Autodesk Inventor part; units mm, degrees
ref_plane "YZ Plane" through (0, 0, 0) normal (1, 0, 0) x (0, 1, 0)
ref_plane "XZ Plane" through (0, 0, 0) normal (0, 1, 0) x (-1, 0, 0)
ref_plane "XY Plane" through (0, 0, 0) normal (0, 0, 1) x (1, 0, 0)
sketch "Sketch1" plane through (0, 0, 0) normal (0, 0, 1) x (1, 0, 0)
  line L0 (-1.5, 81) -> (1.5, 81)
  line L1 (1.5, 81) -> (1.5, 86)
  line L2 (-1.5, 86) -> (1.5, 86)
  line L3 (-1.5, 86) -> (-1.5, 81)
  arc A0 (-53.4049, -82.5) -> (-44.7446, -87.5) centre (-44.7446, -77.5) ccw
  line L4 (-44.7446, -87.5) -> (44.7446, -87.5)
  arc A1 (44.7446, -87.5) -> (53.4049, -82.5) centre (44.7446, -77.5) ccw
  line L5 (53.4049, -82.5) -> (98.1495, -5)
  arc A2 (98.1495, -5) -> (98.1495, 5) centre (89.4893, 0) ccw
  line L6 (98.1495, 5) -> (53.4049, 82.5)
  arc A3 (53.4049, 82.5) -> (44.7446, 87.5) centre (44.7446, 77.5) ccw
  line L7 (44.7446, 87.5) -> (-44.7446, 87.5)
  arc A4 (-44.7446, 87.5) -> (-53.4049, 82.5) centre (-44.7446, 77.5) ccw
  line L8 (-53.4049, 82.5) -> (-98.1495, 5)
  arc A5 (-98.1495, 5) -> (-98.1495, -5) centre (-89.4893, 0) ccw
  line L9 (-98.1495, -5) -> (-53.4049, -82.5)
  line L10 (-50.8068, -84) -> (-98.1495, -2)
  arc A6 (-98.1495, 2) -> (-98.1495, -2) centre (-94.6854, 0) ccw
  line L11 (-98.1495, 2) -> (-50.8068, 84)
  arc A7 (-47.3427, 86) -> (-50.8068, 84) centre (-47.3427, 82) ccw
  line L12 (-47.3427, 86) -> (47.3427, 86)
  arc A8 (50.8068, 84) -> (47.3427, 86) centre (47.3427, 82) ccw
  line L13 (50.8068, 84) -> (98.1495, 2)
  arc A9 (98.1495, -2) -> (98.1495, 2) centre (94.6854, 0) ccw
  line L14 (98.1495, -2) -> (50.8068, -84)
  arc A10 (47.3427, -86) -> (50.8068, -84) centre (47.3427, -82) ccw
  line L15 (47.3427, -86) -> (-47.3427, -86)
  arc A11 (-50.8068, -84) -> (-47.3427, -86) centre (-47.3427, -82) ccw
  line L16 (47.3427, 89) -> (-47.3427, 89)
  line L17 (1.5, 94) -> (-1.5, 94)
  line L18 (-1.5, 94) -> (-1.5, 89)
  line L19 (1.5, 89) -> (-1.5, 89)
  line L20 (1.5, 89) -> (1.5, 94)
  line L21 (1.5, 97) -> (1.5, 94)
  line L22 (-1.5, 97) -> (1.5, 97)
  line L23 (-1.5, 94) -> (-1.5, 97)
  line L24 (1.5, 94) -> (-1.5, 94)
  line L25 (-1.5, 78) -> (-1.5, 81)
  line L26 (1.5, 78) -> (-1.5, 78)
  line L27 (1.5, 81) -> (1.5, 78)
  line L28 (-1.5, 81) -> (1.5, 81)
  line L29 (-11.5, 89) -> (11.5, 89)
  line L30 (11.5, 89) -> (11.5, 86)
  line L31 (11.5, 86) -> (-11.5, 86)
  line L32 (-11.5, 86) -> (-11.5, 89)
  line L33 (1.5, 92) -> (1.5, 83)
  line L34 (-1.5, 83) -> (-1.5, 92)
  line L35 (1.5, 92) -> (-1.5, 92)
  line L36 (1.5, 83) -> (-1.5, 83)
  point P0 (0, 0)
  dimension "d0" = 10
  dimension "d1" = 10
  dimension "d14" = 3
  dimension "d15" = 3
extrude "Extrusion1" add sketch "Sketch1" along normal blind 4 contours L3 L36 L1 L0 | L3 L2 L1 L36 | L34 L7 L33 L2 | L12 L32 L7 L34 | L33 L7 L30 L12 | L34 L16 L33 L7 | L7 L32 L16 L34 | L33 L16 L30 L7 | L18 L35 L20 L16 | L18 L17 L20 L35
sketch "Sketch2" plane through (0, 0, 4) normal (0, 0, 1) x (1, 0, 0)
  line L0 (1.5, 81) -> (1.5, 86)
  line L1 (1.5, 86) -> (11.5, 86)
  line L2 (11.5, 86) -> (11.5, 89)
  line L3 (11.5, 89) -> (1.5, 89)
  line L4 (1.5, 89) -> (1.5, 94)
  line L5 (-1.5, 94) -> (-1.5, 89)
  line L6 (-1.5, 89) -> (-11.5, 89)
  line L7 (-11.5, 89) -> (-11.5, 86)
  line L8 (-11.5, 86) -> (-1.5, 86)
  line L9 (-1.5, 86) -> (-1.5, 81)
  line L10 (-1.5, 81) -> (1.5, 81)
  line L11 (1.5, 94) -> (-1.5, 94)
  point P0 (0, 0)
sketch "Sketch3" plane through (0, 0, 4) normal (0, 0, 1) x (1, 0, 0)
  line L0 (11.5, 92) -> (-11.5, 92)
  line L1 (-11.5, 92) -> (-11.5, 83)
  line L2 (-11.5, 83) -> (11.5, 83)
  line L3 (11.5, 83) -> (11.5, 92)
  line L4 (11.5, 86) -> (11.5, 89)
  line L5 (-11.5, 89) -> (-11.5, 86)
  line L6 (1.5, 86) -> (11.5, 86)
  line L7 (11.5, 89) -> (1.5, 89)
  line L8 (-1.5, 86) -> (-11.5, 86)
  line L9 (-11.5, 86) -> (-11.5, 83)
  line L10 (-11.5, 83) -> (-1.5, 83)
  line L11 (-1.5, 83) -> (-1.5, 86)
  line L12 (-11.5, 89) -> (-11.5, 86)
  line L13 (-1.5, 92) -> (-11.5, 92)
  line L14 (-11.5, 92) -> (-11.5, 89)
  line L15 (-11.5, 89) -> (-1.5, 89)
  line L16 (-1.5, 89) -> (-1.5, 92)
  line L17 (-1.5, 94) -> (-1.5, 89)
  line L18 (1.5, 81) -> (1.5, 86)
  line L19 (11.5, 83) -> (1.5, 83)
  line L20 (1.5, 83) -> (1.5, 86)
  line L21 (1.5, 86) -> (11.5, 86)
  line L22 (11.5, 86) -> (11.5, 83)
  line L23 (11.5, 89) -> (1.5, 89)
  line L24 (1.5, 89) -> (1.5, 92)
  line L25 (1.5, 92) -> (11.5, 92)
  line L26 (11.5, 92) -> (11.5, 89)
  point P0 (0, 0)
  point P1 (-1.5, 97)
  point P2 (1.5, 78)
  dimension "d4" = 3
  dimension "d5" = 3
extrude "Extrusion2" add sketch "Sketch3" against normal blind 15 contours L3 L7 L24 L0 | L16 L15 L1 L0 | L3 L2 L18 L6 | L8 L11 L2 L1
sketch "Sketch4" plane through (0, 0, 0) normal (0, 0, -1) x (-1, 0, 0)
  line L0 (-1.5, 89) -> (-1.5, 92)
  line L1 (-11.5, 89) -> (-1.5, 89)
  line L2 (-11.5, 86) -> (-11.5, 89)
  line L3 (-1.5, 86) -> (-11.5, 86)
  line L4 (-1.5, 83) -> (-1.5, 86)
  line L5 (-1.5, 81) -> (-1.5, 83)
  line L6 (1.5, 83) -> (1.5, 81)
  line L7 (1.5, 86) -> (1.5, 83)
  line L8 (11.5, 86) -> (1.5, 86)
  line L9 (11.5, 89) -> (11.5, 86)
  line L10 (1.5, 89) -> (11.5, 89)
  line L11 (1.5, 92) -> (1.5, 89)
  line L12 (1.5, 94) -> (1.5, 92)
  line L13 (-1.5, 92) -> (-1.5, 94)
  line L14 (-1.5, 83) -> (-1.5, 86)
  line L15 (-1.5, 86) -> (-11.5, 86)
  line L16 (-11.5, 86) -> (-11.5, 83)
  line L17 (-11.5, 83) -> (-1.5, 83)
  line L18 (-1.5, 89) -> (-1.5, 92)
  line L19 (-1.5, 92) -> (-11.5, 92)
  line L20 (-11.5, 92) -> (-11.5, 89)
  line L21 (-11.5, 89) -> (-1.5, 89)
  line L22 (1.5, 89) -> (11.5, 89)
  line L23 (11.5, 89) -> (11.5, 92)
  line L24 (11.5, 92) -> (1.5, 92)
  line L25 (1.5, 92) -> (1.5, 89)
  line L26 (11.5, 83) -> (11.5, 86)
  line L27 (11.5, 86) -> (1.5, 86)
  line L28 (1.5, 86) -> (1.5, 83)
  line L29 (1.5, 83) -> (11.5, 83)
  line L30 (-1.5, 89) -> (-1.5, 92)
  line L31 (1.5, 89) -> (-1.5, 89)
  line L32 (-1.5, 89) -> (-1.5, 92)
  line L33 (-1.5, 92) -> (1.5, 92)
  line L34 (1.5, 92) -> (1.5, 89)
  line L35 (-1.5, 83) -> (-1.5, 86)
  line L36 (1.5, 86) -> (-1.5, 86)
  line L37 (-1.5, 86) -> (-1.5, 83)
  line L38 (-1.5, 83) -> (1.5, 83)
  line L39 (1.5, 83) -> (1.5, 86)
  line L40 (1.5, 81) -> (-1.5, 81)
  line L41 (-1.5, 94) -> (1.5, 94)
  point P0 (0, 0)
  dimension "d8" = 3
  dimension "d9" = 3
  dimension "d10" = 3
  dimension "d11" = 3
extrude "Extrusion3" add sketch "Sketch4" along normal blind 3 contours L0 L33 L11 L31 | L36 L7 L38 L4
equation "\"d1\" = d0"
equation "\"d15\" = d14"
equation "\"d5\" = d4"
properties part number "Aligner Helper v1"
CAD build for the part. Positions are in the model's coordinates, mm. A direction names the side the tool comes from. Give positions to 0.01 mm unless a question says otherwise; leave off trailing zeros. Loops run counter-clockwise (first coordinate to the right, second up) from the corner with the lowest first, then second, coordinate; pieces in that order, holes last. Notation, with made-up numbers: M 49,-31.75 L 66,-31.75 A20 ccw 66,-4.75 Z; hole C 61.5,-31.75 d4. An arc over 180 degrees is marked long. Write each question's results on one line, items separated by ' | '.
Q1. Flat gauge pins, fed straight in: P1, Ø1.5, axis at x = -5.5, z = 2.5, coming from the -Y side; P2, Ø1, axis at y = 93, z = 1, coming from the -X side; P3, Ø9, axis at x = -5.5, z = -4.5, coming from the +Y side; P4, Ø3.5, axis at x = -0.5, y = 91, coming from the -Z side. Where does each tip first touch, or does it go through?
Geometry check:
P1: stops at y = 83 | P2: stops at x = -1.5 | P3: stops at y = 92 | P4: stops at z = -11
Q2. Band-saw the part on D-D on y = 85. Write the cut outline in (x, z), and give its area (3 significant figures).
Geometry check:
outline: M -11.5,-11 L -1.5,-11 L -1.5,-3 L 1.5,-3 L 1.5,-11 L 11.5,-11 L 11.5,4 L -11.5,4 Z | area: 321 mm²
Q3. Band-saw the part on C-C on x = 0. Write the cut outline in (y, z).
Geometry check:
outline: M 81,0 L 83,0 L 83,-3 L 86,-3 L 86,0 L 89,0 L 89,-3 L 92,-3 L 92,0 L 94,0 L 94,4 L 81,4 Z
Q4. Probe probe 1 along Y at (x, z) = (-3.5, -8.25); probe 2 along X at (y, z) = (85.25, -9); probe 3 along Z at (x, y) = (2.75, 88). List the from-to ranges inside material, lowest first.
Geometry check:
probe 1: y = 83 to 86, 89 to 92 | probe 2: x = -11.5 to -1.5, 1.5 to 11.5 | probe 3: z = 0 to 4
Q5. Band-saw the part on A-A on z = -9.25. Write the cut outline in (x, y), and give its area (3 significant figures).
Geometry check:
outline: M -11.5,83 L -1.5,83 L -1.5,86 L -11.5,86 Z; M -11.5,89 L -1.5,89 L -1.5,92 L -11.5,92 Z; M 1.5,83 L 11.5,83 L 11.5,86 L 1.5,86 Z; M 1.5,89 L 11.5,89 L 11.5,92 L 1.5,92 Z | area: 120 mm²
Q6. Mould opens along Y. For faces 4 (the face through (0, 81, 2)), 5 (the face through (-11.5, 85, -4)), 6 (the face through (-3, 86, -5)) say: pulls with the +Y half, pulls with the -Y half, needs draft (parallel to the pull), parting line crosses it, or undercut.
Geometry check:
face 4: pulls with the -Y half | face 5: needs draft | face 6: undercut
Q7. Band-saw the part on B-B on z = -0.5. Write the cut outline in (x, y), and give its area (3 significant figures).
Geometry check:
outline: M -11.5,83 L 11.5,83 L 11.5,86 L -11.5,86 Z; M -11.5,89 L 11.5,89 L 11.5,92 L -11.5,92 Z | area: 138 mm²
Q8. Which spindle directions (+Z, -Z, +X, -X, +Y, -Y) get a long thin tool onto all of the face, cutting with end or side? Do faces 1 (the face through (-1.5, 82, 2)), 2 (the face through (1.5, 84, -7)), 3 (the face through (0, 93, 0)). Say none if no direction does.
Geometry check:
face 1: +Z, -Z, -X, -Y | face 2: -Z, +Y, -Y | face 3: -Z, +X, -X, +Y
